Build history of the part. All positions in model axes, mm. A direction names the side the tool comes from. Round coordinates to 2 decimals unless told otherwise and drop trailing zeros. Loops run counter-clockwise (first coordinate to the right, second up) from the corner with the lowest first, then second, coordinate; pieces in that order, holes last. Notation, with made-up numbers: (76.5, 18.5) -> (126.5, 18.5) arc R16 ccw to (126.5, 38.5) -> close; hole circle Ø8 at (66, 31.25). An arc over 180 degrees is marked (long way). Put each result on its own line as item: value. Start each with the question number.
```python
from build123d import *

# Parameters (mm, degrees)
SKETCH1_R           = 26.5
BOSS_EXTRUDE1_DEPTH = 230
SKETCH2_R           = 26.5
SKETCH2_R_2         = 11.564416293
CUT_EXTRUDE1_DEPTH  = 25.4
FILLET1_R           = 20
FILLET2_R           = 50
FILLET3_R           = 10
SKETCH3_W           = 6.947530086
SKETCH3_H           = 7.989839498
BOSS_EXTRUDE2_DEPTH = 5.4
SKETCH4_R           = 1.894960562
BOSS_EXTRUDE3_DEPTH = 15.4


with BuildPart() as part:
    # Sketch1 → Boss-Extrude1 (new body)
    with BuildSketch(Plane(origin=(0, 0, 0), x_dir=(1, 0, 0), z_dir=(0, 1, 0))):
        with Locations(Location((0, 0, 0), (0, 0, 270))):
            Circle(SKETCH1_R)
    extrude(amount=BOSS_EXTRUDE1_DEPTH)

    # Sketch2 → Cut-Extrude1 (cut)
    with BuildSketch(Plane.XZ):
        with Locations(Location((0, 0, 0), (0, 0, 270))):
            Circle(SKETCH2_R)
        with Locations(Location((0, 0, 0), (0, 0, 270))):
            Circle(SKETCH2_R_2, mode=Mode.SUBTRACT)
    extrude(amount=-CUT_EXTRUDE1_DEPTH, mode=Mode.SUBTRACT)

    # Fillet1
    # the kernel refuses this fillet: 20 mm, written as the material it takes off along each edge
    with BuildSketch(Plane(origin=(0, 25.4, 0), x_dir=(0, 0, 1), z_dir=(-1, 0, 0))) as fillet1_piece_1:
        with BuildLine():
            CenterArc((6.5, 19.348170136), FILLET1_R, 284.668185606, 75.331814394)
            Line((11.564416293, 0), (11.665704619, -0.386963403))
            ThreePointArc((11.665704619, -0.386963403), (19.032208147, -0.4), (26.5, -0.4))
            Line((26.5, -0.4), (26.9, 0))
            Line((26.9, 0), (26.9, 19.348170136))
            Line((26.9, 19.348170136), (26.5, 19.348170136))
        make_face()
    revolve(axis=Axis((0, 25.4, 0), (0, 1, 0)), mode=Mode.SUBTRACT)

    # Fillet2
    fillet2_edges = [part.edges().sort_by_distance(p)[0] for p in [
        (11.564416293, 25.4, 0),
    ]]
    fillet(fillet2_edges, radius=FILLET2_R)

    # Fillet3
    fillet3_edges = [part.edges().sort_by_distance(p)[0] for p in [
        (0, 230, -26.5),
    ]]
    fillet(fillet3_edges, radius=FILLET3_R)

    # Sketch3 → Boss-Extrude2 (add)
    with BuildSketch(Plane.XZ):
        Rectangle(SKETCH3_W, SKETCH3_H)
    extrude(amount=BOSS_EXTRUDE2_DEPTH)

    # Sketch4 → Boss-Extrude3 (add)
    with BuildSketch(Plane(origin=(0, -5.4, 0), x_dir=(-1, 0, 0), z_dir=(0, -1, 0))):
        with Locations(Location((0, 0, 0), (0, 0, 90))):
            Circle(SKETCH4_R)
    extrude(amount=BOSS_EXTRUDE3_DEPTH)


solid = part.part
```
Item 1: Drop flat-ended pins along their axis: pin 1 (6 mm diameter, centred on y = 112.5, z = 18, fed in from -X); pin 2 (1 mm diameter, centred on y = 103.5, z = 9, fed in from -X); pin 3 (4 mm diameter, centred on y = 190, z = 18, fed in from +X). Give the stop position or say it passes through.
Item 2: Wall check: line 1 (Y direction, x = 7.5, z = 7.5); line 2 (Z direction, x = 1, y = 120). Give the ranges that are in metal, low to high. Write a range as from..to.
Item 3: 3-axis set-ups, long thin cutter, end or side, ignore diameter. For faces 1 (the face through (3.474, -3, 0)), 2 (the face through (-11.29, 0.75, 2.51)), 3 (the face through (0, -3, -3.995)), 4 (the face through (0, -3, 3.995)): which of +Z, -Z, +X, -X, +Y, -Y reach the whole face in a straight line?
Item 4: Cut at A-A on y = 146. Write the cut outline in (x, z), then the cut area to 3 significant figures.
Ans:
1. pin 1: stops at x = -21.85
1. pin 2: stops at x = -25.1
1. pin 3: stops at x = 21.12
2. line 1: y = 0..230
2. line 2: z = -26.48..26.48
3. face 1: +Z, -Z, +X, -Y
3. face 2: -Y
3. face 3: -Z, +X, -X, -Y
3. face 4: +Z, +X, -X, -Y
4. outline: circle Ø53 at (0, 0)
4. area: 2,210 mm2
